from build123d import *

# Parameters (mm, degrees)
SKETCH1_W           = 77.51
SKETCH1_H           = 77.519
SKETCH1_R           = 2.55
BOSS_EXTRUDE1_DEPTH = 6
CUT_EXTRUDE1_DEPTH  = 6
FILLET1_R           = 4.635
CUT_EXTRUDE2_DEPTH  = 1.5
SKETCH4_R           = 4.5
SKETCH4_R_2         = 6
CUT_EXTRUDE3_DEPTH  = 1.5
SKETCH5_R           = 3.6
CUT_EXTRUDE4_DEPTH  = 7


with BuildPart() as part:
    # Sketch1 → Boss-Extrude1 (new body)
    with BuildSketch(Plane.XY):
        Rectangle(SKETCH1_W, SKETCH1_H)
        with Locations((-30.05, 30.0005)):
            Circle(SKETCH1_R, mode=Mode.SUBTRACT)
        with Locations((-10.05, 30.0005)):
            Circle(SKETCH1_R, mode=Mode.SUBTRACT)
        with Locations((-10.05, -29.9995)):
            Circle(SKETCH1_R, mode=Mode.SUBTRACT)
        with Locations((0, 20)):
            Circle(SKETCH1_R, mode=Mode.SUBTRACT)
        with Locations((0, 10)):
            Circle(SKETCH1_R, mode=Mode.SUBTRACT)
        with Locations((-10.05, 10)):
            Circle(SKETCH1_R, mode=Mode.SUBTRACT)
        with Locations((9.95, 30.0005)):
            Circle(SKETCH1_R, mode=Mode.SUBTRACT)
        with Locations((9.95, -29.9995)):
            Circle(SKETCH1_R, mode=Mode.SUBTRACT)
        with Locations((-10.05, -10)):
            Circle(SKETCH1_R, mode=Mode.SUBTRACT)
        with Locations((9.95, 0.0005)):
            Circle(SKETCH1_R, mode=Mode.SUBTRACT)
        with Locations((-30.05, -29.9995)):
            Circle(SKETCH1_R, mode=Mode.SUBTRACT)
        with Locations((-30.05, -14.2495)):
            Circle(SKETCH1_R, mode=Mode.SUBTRACT)
        with Locations((-30.05, 0.0005)):
            Circle(SKETCH1_R, mode=Mode.SUBTRACT)
        with Locations((-30.05, 14.2505)):
            Circle(SKETCH1_R, mode=Mode.SUBTRACT)
        with Locations((0, -10)):
            Circle(SKETCH1_R, mode=Mode.SUBTRACT)
        with Locations((29.95, 30.0005)):
            Circle(SKETCH1_R, mode=Mode.SUBTRACT)
        with Locations((29.95, -29.9995)):
            Circle(SKETCH1_R, mode=Mode.SUBTRACT)
        with Locations((29.95, -14.2495)):
            Circle(SKETCH1_R, mode=Mode.SUBTRACT)
        with Locations((29.95, 0.0005)):
            Circle(SKETCH1_R, mode=Mode.SUBTRACT)
        with Locations((29.95, 14.2505)):
            Circle(SKETCH1_R, mode=Mode.SUBTRACT)
        with Locations((0, -20)):
            Circle(SKETCH1_R, mode=Mode.SUBTRACT)
        with Locations((20, 20)):
            Circle(SKETCH1_R, mode=Mode.SUBTRACT)
        with Locations((20, 10)):
            Circle(SKETCH1_R, mode=Mode.SUBTRACT)
        with Locations((20, -10)):
            Circle(SKETCH1_R, mode=Mode.SUBTRACT)
        with Locations((20, -20)):
            Circle(SKETCH1_R, mode=Mode.SUBTRACT)
        with Locations((-20, 20)):
            Circle(SKETCH1_R, mode=Mode.SUBTRACT)
        with Locations((-20, 10)):
            Circle(SKETCH1_R, mode=Mode.SUBTRACT)
        with Locations((-20, -10)):
            Circle(SKETCH1_R, mode=Mode.SUBTRACT)
        with Locations((-20, -20)):
            Circle(SKETCH1_R, mode=Mode.SUBTRACT)
    extrude(amount=BOSS_EXTRUDE1_DEPTH)

    # Sketch2 → Cut-Extrude1 (cut)
    with BuildSketch(Plane.XY.offset(6)):
        with BuildLine():
            Line((-10.049999987, 2.55), (-0.049999987, 2.55))
            ThreePointArc((-0.049999987, 2.55), (2.500000013, 0), (-0.049999987, -2.55))
            Line((-0.049999987, -2.55), (-10.049999987, -2.55))
            ThreePointArc((-10.049999987, -2.55), (-12.599999987, 0), (-10.049999987, 2.55))
        make_face()
    extrude(amount=-CUT_EXTRUDE1_DEPTH, mode=Mode.SUBTRACT)

    # Fillet1
    fillet1_edges = [part.edges().sort_by_distance(p)[0] for p in [
        (-38.755, 38.7595, 3),
        (38.755, 38.7595, 3),
        (38.755, -38.7595, 3),
        (-38.755, -38.7595, 3),
    ]]
    fillet(fillet1_edges, radius=FILLET1_R)

    # Sketch3 → Cut-Extrude2 (cut)
    with BuildSketch(Plane.XY.offset(6)):
        with BuildLine():
            Line((-10.03, 14.05), (10.03, 14.05))
            ThreePointArc((10.03, 14.05), (13.50967247, 12.60867247), (14.951, 9.129))
            Line((14.951, 9.129), (14.951, -10.029))
            ThreePointArc((14.951, -10.029), (13.50967247, -13.50867247), (10.03, -14.95))
            Line((10.03, -14.95), (-10.03, -14.95))
            ThreePointArc((-10.03, -14.95), (-13.50967247, -13.50867247), (-14.951, -10.029))
            Line((-14.951, -10.029), (-14.951, 9.129))
            ThreePointArc((-14.951, 9.129), (-13.50967247, 12.60867247), (-10.03, 14.05))
        make_face()
    extrude(amount=-CUT_EXTRUDE2_DEPTH, mode=Mode.SUBTRACT)

    # Sketch4 → Cut-Extrude3 (cut)
    with BuildSketch(Plane.XY.offset(6)):
        with Locations((-30.05, -14.2495)):
            Circle(SKETCH4_R)
        with Locations((29.95, -14.2495)):
            Circle(SKETCH4_R)
        with Locations((-30.05, 14.2505)):
            Circle(SKETCH4_R_2)
        with Locations((29.95, 14.2505)):
            Circle(SKETCH4_R_2)
    extrude(amount=-CUT_EXTRUDE3_DEPTH, mode=Mode.SUBTRACT)

    # Sketch5 → Cut-Extrude4 (cut, through all)
    with BuildSketch(Plane.XY.offset(6)):
        with Locations((-30.05, 14.2505)):
            Circle(SKETCH5_R)
        with Locations((29.95, 14.2505)):
            Circle(SKETCH5_R)
    extrude(amount=-CUT_EXTRUDE4_DEPTH, mode=Mode.SUBTRACT)


solid = part.part
Model file for the job. Use its own axes, mm. A direction names the side the tool comes from. Give positions to 0.01 mm unless a question says otherwise; leave off trailing zeros. Loops run counter-clockwise (first coordinate to the right, second up) from the corner with the lowest first, then second, coordinate; pieces in that order, holes last. Notation, with made-up numbers: (-30, -15) - (2, -15) arc R16 cw to (2, 12) - close; hole circle Ø5 at (64.5, 28.5). An arc over 180 degrees is marked (long way). Use one line per item in the form item = value.
(1) Drill centre lines: L1, parallel to Y at x = 9.95, z = 3.8; L2, parallel to Y at x = 29.95, z = 5.2; L3, parallel to Y at x = -30, z = 1.9. Where is each one in solid material? Low to high.
Determined:
L1 = -38.76 to -32.55, -27.45 to -2.55, 2.55 to 27.45, 32.55 to 38.76
L2 = -38.76 to -32.55, -27.45 to -18.75, -9.75 to -2.55, 2.55 to 8.25, 20.25 to 27.45, 32.55 to 38.76
L3 = -38.76 to -32.55, -27.45 to -16.8, -11.7 to -2.55, 2.55 to 10.65, 17.85 to 27.45, 32.55 to 38.76
(2) Cut at C-C (x = 21). Give the cut face in (y, z), then the cut area to 3 significant figures.
Determined:
outline = (-38.76, 0) - (-22.35, 0) - (-22.35, 6) - (-38.76, 6) - close; (-17.65, 0) - (-12.35, 0) - (-12.35, 6) - (-17.65, 6) - close; (-7.65, 0) - (7.65, 0) - (7.65, 6) - (-7.65, 6) - close; (12.35, 0) - (17.65, 0) - (17.65, 6) - (12.35, 6) - close; (22.35, 0) - (38.76, 0) - (38.76, 6) - (22.35, 6) - close
area = 353 mm^2
(3) Pull direction X, two halves, no side cores. Call faces 1 (the face through (0, -38.76, 3)), 2 (the face through (-37.4, -37.4, 3)), 3 (the face through (1.18, 17.74, 2.96)): pulls with the +X half, pulls with the -X half, needs draft (parallel to the pull), parting line crosses it, or undercut.
Determined:
face_1 = needs draft
face_2 = pulls with the -X half
face_3 = undercut
(4) Cut at B-B (y = 6). Give the cut face in (x, z) (3 decimals), then the cut area to 3 significant figures.
Determined:
outline = (-38.755, 0) - (38.755, 0) - (38.755, 6) - (14.951, 6) - (14.951, 4.5) - (-14.951, 4.5) - (-14.951, 6) - (-38.755, 6) - close
area = 420 mm^2
(5) Drop a flat-ended pin along its axis: P1, Ø8.5, axis at x = -1, y = 0.5, coming from the +Z side. Give the stop position or say it passes through.
Determined:
P1 = 4.5
(6) Cut at A-A (y = -20). Give the cut face in (x, z) (3 decimals), then the cut area to 3 significant figures.
Determined:
outline = (-38.755, 0) - (-22.55, 0) - (-22.55, 6) - (-38.755, 6) - close; (-17.45, 0) - (-2.55, 0) - (-2.55, 6) - (-17.45, 6) - close; (2.55, 0) - (17.45, 0) - (17.45, 6) - (2.55, 6) - close; (22.55, 0) - (38.755, 0) - (38.755, 6) - (22.55, 6) - close
area = 373 mm^2
(7) Cut at D-D (x = 1). Give the cut face in (y, z).
Determined:
outline = (-38.76, 0) - (-22.35, 0) - (-22.35, 6) - (-38.76, 6) - close; (-17.65, 0) - (-12.35, 0) - (-12.35, 4.5) - (-14.95, 4.5) - (-14.95, 6) - (-17.65, 6) - close; (-7.65, 0) - (-2.32, 0) - (-2.32, 4.5) - (-7.65, 4.5) - close; (2.32, 0) - (7.65, 0) - (7.65, 4.5) - (2.32, 4.5) - close; (12.35, 0) - (17.65, 0) - (17.65, 6) - (14.05, 6) - (14.05, 4.5) - (12.35, 4.5) - close; (22.35, 0) - (38.76, 0) - (38.76, 6) - (22.35, 6) - close
(8) 3-axis set-ups, long thin cutter, end or side, ignore diameter. For faces 4 (the face through (0, -3, 4.5)), 5 (the face through (-22.024, -11.552, 2.958)): which of +Z, -Z, +X, -X, +Y, -Y reach the whole face in a straight line?
Determined:
face_4 = +Z
face_5 = +Z, -Z
